Check sheet for the modelled part. Datum: model origin and axes. Units: mm. A direction names the side the tool comes from. Round coordinates to 2 decimals unless told otherwise and drop trailing zeros. Write each loop counter-clockwise with the first axis right and the second up, starting at its lowest first coordinate (ties: lowest second). Pieces come first, ordered by that corner, then holes. Notation, with made-up numbers: M -21,48 L 21,48 A14 cw 21,61 Z; hole C -27.5,64.25 d3. An arc over 180 degrees is marked long. Put each result on its own line as item: value.
```python
from build123d import *

# Parameters (mm, degrees)
BOSS_EXTRUDE1_DEPTH = 95
SKETCH3_R           = 41.5
BOSS_EXTRUDE3_DEPTH = 45


with BuildPart() as part:
    # Sketch2 → Boss-Extrude1 (new body, symmetric)
    with BuildSketch(Plane(origin=(0, 0, 0), x_dir=(1, 0, 0), z_dir=(0, 1, 0))):
        Polygon((-84.852813742, 0), (0, -84.852813742), (84.852813742, 0), (0, 84.852813742), align=None)
    extrude(amount=BOSS_EXTRUDE1_DEPTH, both=True)

    # Sketch3 → Boss-Extrude3 (add)
    with BuildSketch(Plane.XY.offset(84.852813742)):
        with Locations((0, -13.5)):
            Circle(SKETCH3_R)
    extrude(amount=-BOSS_EXTRUDE3_DEPTH)


solid = part.part
```
1. Cross-section at A-A (y = -13.5). Enter the section's corners in (x, z).
Computed values:
outline: M -84.85,0 L 0,-84.85 L 84.85,0 L 41.5,43.35 L 41.5,84.85 L -41.5,84.85 L -41.5,43.35 Z
2. Cross-section at D-D (y = -43). Enter the section's corners in (x, z), then the cut area to 3 significant figures.
Computed values:
outline: M -84.85,0 L 0,-84.85 L 84.85,0 L 29.19,55.66 L 29.19,84.85 L -29.19,84.85 L -29.19,55.66 Z
area: 15,300 mm2
3. Access from +Z, -Z, +X, -X, +Y, -Y to the whole of each face (thin tool, end or side, straight path). Record for faces 1 (the flat face through (-52.45, 1.33, 32.4)), 2 (the flat face through (51.26, 1.33, 33.59)), 3 (the flat face through (-1, -95, -1)).
Computed values:
face 1: +Z, -X
face 2: +Z, +X
face 3: +Z, -Z, +X, -X, -Y
4. Depth check by flat-ended pin: pin 1 Ø5 at (y, z) = (51.5, -33) entering from -X; pin 2 Ø5 at (x, y) = (67.5, 4) entering from +Z; pin 3 Ø2 at (x, z) = (36, 53) entering from +Y. Enter the tip coordinate at first touch or a pass-through.
Computed values:
pin 1: stops at x = -54.35
pin 2: stops at z = 19.85
pin 3: stops at y = 8.8
5. Cross-section at C-C (z = 56). Enter the section's corners in (x, y), then the cut area to 3 significant figures.
Computed values:
outline: M -28.85,-95 L 28.85,-95 L 28.85,-43.33 A41.5 ccw 28.85,16.33 L 28.85,95 L -28.85,95 L -28.85,16.33 A41.5 ccw -28.85,-43.33 Z
area: 12,000 mm2
6. Scan lines: probe 1 along X at (y, z) = (83.5, 50); probe 2 along Z at (x, y) = (66, 3.5); probe 3 along X at (y, z) = (33, -26). Record each from-to range of solid material in increasing order.
Computed values:
probe 1: x = -34.85 to 34.85
probe 2: z = -18.85 to 18.85
probe 3: x = -58.85 to 58.85
7. Cross-section at B-B (x = 29). Enter the section's corners in (y, z).
Computed values:
outline: M -95,-55.85 L 95,-55.85 L 95,55.85 L 16.19,55.85 L 16.19,84.85 L -43.19,84.85 L -43.19,55.85 L -95,55.85 Z
